Geometry: final body of the model. Coordinates: model frame, mm. A direction names the side the tool comes from. Give positions to 0.01 mm unless a question says otherwise; leave off trailing zeros. Write each loop counter-clockwise with the first axis right and the second up, starting at its lowest first coordinate (ties: lowest second). Pieces come first, ordered by that corner, then holes. Notation, with made-up numbers: (54.5, 80.5) -> (102.5, 80.5) arc R11 cw to (102.5, 94.5) -> close; hole circle Ø11 at (-40, 52). An arc over 180 degrees is marked (long way). Answer in a Markdown table with one row per item. Add a question column.
Item 1: Draft query along X for faces 1 (the flat face through (26, 0, 1)), 2 (the flat face through (1.74, 12.79, 1.19)), 3 (the cylindrical face through (41.433, 9.438, 1.002)), 4 (the cylindrical face through (23.787, 9.045, 1.002)). Return one class per face: +X half, -X half, draft (parallel to the pull), parting line (faces both ways), or undercut.
Item 2: Section query B-B on z = -3.5. Output: boundary loops of the cut face in (x, y) (3 decimals), plus the area to 3 significant figures.
Item 3: Material intervals for probe 1 along Y at (x, z) = (18.5, 1.5); probe 2 along Z at (x, y) = (49.5, 1.75); probe 3 along Z at (x, y) = (33, 7.75), sorted ascending. Write a range as from..to.
Item 4: First-contact query: P1, Ø6, axis at x = 34, y = 13, coming from the +Z side; P2, Ø2.5, axis at x = 27.813, y = 9.398, coming from the -Z side; P3, Ø1.5, axis at x = 40.513, y = 9.398, coming from the -Z side; P4, Ø1.2, axis at x = 30.5, z = -1.5, coming from the -Y side. Flat tips, straight axial feed; report the tip coordinate or a pass-through.
Item 5: Section query A-A on x = 12. Output: boundary loops of the cut face in (y, z).
Item 6: Access query for faces 5 (the flat face through (52.324, 7, 1)), 6 (the cylindrical face through (48.996, 6.188, 1.19)). Directions: +Z, -Z, +X, -X, +Y, -Y. A direction counts if a zero-diameter tool reaches every point of the face in a straight line with its end or side. Return the directions, or none.
Item 7: Section query C-C on z = 0.75. State how many separate pieces and enclosed holes the cut face has, plus the area to 3 significant figures.
```python
from build123d import *

# Parameters (mm, degrees)
BOSS_EXTRUDE1_DEPTH = 2.032
BOSS_EXTRUDE2_DEPTH = 0.381
SKETCH3_W           = 45.466
SKETCH3_H           = 1.524
BOSS_EXTRUDE3_DEPTH = 4.064
SKETCH4_R           = 1.6129
SKETCH4_R_2         = 0.92075
CUT_EXTRUDE1_DEPTH  = 55.441983395


with BuildPart() as part:
    # Sketch1 → Boss-Extrude1 (new body)
    with BuildSketch(Plane.XY):
        Polygon((0, 3.429), (0, 11.049), (3.429, 14.478), (48.895, 14.478), (52.324, 11.049), (52.324, 3.429), (48.895, 0), (3.429, 0), align=None)
    extrude(amount=BOSS_EXTRUDE1_DEPTH)

    # Sketch2 → Boss-Extrude2 (add)
    with BuildSketch(Plane.XY.offset(2.032)):
        Polygon((0, 11.049), (0, 3.429), (3.429, 0), (10.033, 0), (10.033, 14.478), (3.429, 14.478), align=None)
        Polygon((42.291, 14.478), (42.291, 0), (48.895, 0), (52.324, 3.429), (52.324, 11.049), (48.895, 14.478), align=None)
    extrude(amount=BOSS_EXTRUDE2_DEPTH)

    # Sketch3 → Boss-Extrude3 (add)
    with BuildSketch(Plane(origin=(0, 0, 0), x_dir=(-1, 0, 0), z_dir=(0, 0, -1))):
        with Locations((-26.162, 13.716)):
            Rectangle(SKETCH3_W, SKETCH3_H)
    extrude(amount=BOSS_EXTRUDE3_DEPTH)

    # Sketch4 → Cut-Extrude1 (cut, through all)
    with BuildSketch(Plane(origin=(0, 0, 0), x_dir=(-1, 0, 0), z_dir=(0, 0, -1))):
        with Locations((-5.588, 6.223)):
            Circle(SKETCH4_R)
        with Locations((-11.938, 3.048)):
            Circle(SKETCH4_R_2)
        with Locations((-15.113, 3.048)):
            Circle(SKETCH4_R_2)
        with Locations((-18.288, 3.048)):
            Circle(SKETCH4_R_2)
        with Locations((-21.463, 3.048)):
            Circle(SKETCH4_R_2)
        with Locations((-24.638, 3.048)):
            Circle(SKETCH4_R_2)
        with Locations((-27.813, 3.048)):
            Circle(SKETCH4_R_2)
        with Locations((-30.988, 3.048)):
            Circle(SKETCH4_R_2)
        with Locations((-34.163, 3.048)):
            Circle(SKETCH4_R_2)
        with Locations((-37.338, 3.048)):
            Circle(SKETCH4_R_2)
        with Locations((-40.513, 3.048)):
            Circle(SKETCH4_R_2)
        with Locations((-15.113, 6.223)):
            Circle(SKETCH4_R_2)
        with Locations((-18.288, 6.223)):
            Circle(SKETCH4_R_2)
        with Locations((-21.463, 6.223)):
            Circle(SKETCH4_R_2)
        with Locations((-24.638, 6.223)):
            Circle(SKETCH4_R_2)
        with Locations((-27.813, 6.223)):
            Circle(SKETCH4_R_2)
        with Locations((-30.988, 6.223)):
            Circle(SKETCH4_R_2)
        with Locations((-34.163, 6.223)):
            Circle(SKETCH4_R_2)
        with Locations((-37.338, 6.223)):
            Circle(SKETCH4_R_2)
        with Locations((-40.513, 6.223)):
            Circle(SKETCH4_R_2)
        with Locations((-15.113, 9.398)):
            Circle(SKETCH4_R_2)
        with Locations((-18.288, 9.398)):
            Circle(SKETCH4_R_2)
        with Locations((-21.463, 9.398)):
            Circle(SKETCH4_R_2)
        with Locations((-24.638, 9.398)):
            Circle(SKETCH4_R_2)
        with Locations((-27.813, 9.398)):
            Circle(SKETCH4_R_2)
        with Locations((-30.988, 9.398)):
            Circle(SKETCH4_R_2)
        with Locations((-34.163, 9.398)):
            Circle(SKETCH4_R_2)
        with Locations((-37.338, 9.398)):
            Circle(SKETCH4_R_2)
        with Locations((-40.513, 9.398)):
            Circle(SKETCH4_R_2)
        with Locations((-11.938, 6.223)):
            Circle(SKETCH4_R_2)
        with Locations((-11.938, 9.398)):
            Circle(SKETCH4_R_2)
        with BuildLine():
            Line((-47.3837, 7.8359), (-46.3423, 7.8359))
            ThreePointArc((-46.3423, 7.8359), (-44.7294, 6.223), (-46.3423, 4.6101))
            Line((-46.3423, 4.6101), (-47.3837, 4.6101))
            ThreePointArc((-47.3837, 4.6101), (-48.9966, 6.223), (-47.3837, 7.8359))
        make_face()
    extrude(amount=-CUT_EXTRUDE1_DEPTH, mode=Mode.SUBTRACT)


solid = part.part
```
Findings below:
| question | item | result |
|---|---|---|
| 1 | face 1 | draft |
| 1 | face 2 | -X half |
| 1 | face 3 | undercut |
| 1 | face 4 | undercut |
| 2 | outline | (3.429, 12.954) -> (48.895, 12.954) -> (48.895, 14.478) -> (3.429, 14.478) -> close |
| 2 | area | 69.3 mm^2 |
| 3 | probe 1 | y = 0..2.15, 3.94..5.33, 7.12..8.5, 10.29..14.48 |
| 3 | probe 2 | z = 0..2.41 |
| 3 | probe 3 | z = 0..2.03 |
| 4 | P1 | stops at z = 2.03 |
| 4 | P2 | stops at z = 0 |
| 4 | P3 | passes through |
| 4 | P4 | stops at y = 12.95 |
| 5 | outline | (0, 0) -> (2.13, 0) -> (2.13, 2.03) -> (0, 2.03) -> close; (3.97, 0) -> (5.3, 0) -> (5.3, 2.03) -> (3.97, 2.03) -> close; (7.14, 0) -> (8.48, 0) -> (8.48, 2.03) -> (7.14, 2.03) -> close; (10.32, 0) -> (12.95, 0) -> (12.95, -4.06) -> (14.48, -4.06) -> (14.48, 2.03) -> (10.32, 2.03) -> close |
| 6 | face 5 | +Z, -Z, +X, +Y, -Y |
| 6 | face 6 | +Z, -Z |
| 7 | separate pieces | 1 |
| 7 | enclosed holes | 32 |
| 7 | area | 634 mm^2 |
